```python
from build123d import *

# Parameters (mm, degrees)
BOSS_EXTRUDE2_DEPTH = 5
CUT_EXTRUDE1_DEPTH  = 23.574164436
SKETCH3_W           = 3
SKETCH3_H           = 3.88
BOSS_EXTRUDE3_DEPTH = 12
BOSS_EXTRUDE4_REACH = 35.791
SKETCH4_W           = 3
SKETCH4_H           = 6.078503162
SKETCH6_W           = 3
SKETCH6_H           = 23.7
BOSS_EXTRUDE5_DEPTH = 10.921497
CUT_EXTRUDE2_DEPTH  = 26.634408517
FILLET1_R           = 10
FILLET2_R           = 5


with BuildPart() as part:
    # Sketch1 → Boss-Extrude2 (new body)
    with BuildSketch(Plane(origin=(0, 0, 0), x_dir=(0, 1, 0), z_dir=(0, 0, 1))):
        Polygon((-11.85, 0), (11.85, 0), (11.85, -12.4), (11.85, -15.4), (15.73, -15.4), (15.73, -12.4), (15.73, -0.1), (15.73, 3.9), (-15.73, 3.9), (-15.73, -0.1), (-15.73, -12.4), (-15.73, -15.4), (-11.85, -15.4), (-11.85, -12.4), align=None)
    extrude(amount=BOSS_EXTRUDE2_DEPTH)

    # Sketch2 → Cut-Extrude1 (cut, through all)
    with BuildSketch(Plane.XY.offset(5)):
        with BuildLine():
            Line((4.56, -12.29), (7.06, -12.29))
            ThreePointArc((7.06, -12.29), (8.26, -13.49), (7.06, -14.69))
            Line((7.06, -14.69), (4.56, -14.69))
            ThreePointArc((4.56, -14.69), (3.36, -13.49), (4.56, -12.29))
        make_face()
        with BuildLine():
            Line((4.56, 12.29), (7.06, 12.29))
            ThreePointArc((7.06, 12.29), (8.26, 13.49), (7.06, 14.69))
            Line((7.06, 14.69), (4.56, 14.69))
            ThreePointArc((4.56, 14.69), (3.36, 13.49), (4.56, 12.29))
        make_face()
    extrude(amount=-CUT_EXTRUDE1_DEPTH, mode=Mode.SUBTRACT)

    # Sketch3 → Boss-Extrude3 (add)
    with BuildSketch(Plane(origin=(0, 0, 0), x_dir=(1, 0, 0), z_dir=(0, 0, -1))):
        with Locations((13.9, -13.79)):
            Rectangle(SKETCH3_W, SKETCH3_H)
        with Locations((13.9, 13.79)):
            Rectangle(SKETCH3_W, SKETCH3_H)
    extrude(amount=BOSS_EXTRUDE3_DEPTH)

    # Sketch4 → Boss-Extrude4 (add, up to next)
    with BuildSketch(Plane(origin=(0, -11.85, 0), x_dir=(-1, 0, 0), z_dir=(0, 1, 0)), mode=Mode.PRIVATE) as boss_extrude4_sk1:
        with Locations((-13.9, -8.960748419)):
            Rectangle(SKETCH4_W, SKETCH4_H)
    boss_extrude4_tool1 = extrude(boss_extrude4_sk1.sketch, amount=BOSS_EXTRUDE4_REACH, mode=Mode.PRIVATE) - part.part
    add(boss_extrude4_tool1.solids().sort_by_distance((13.9, -11.85, -8.960748))[0])

    # Sketch6 → Boss-Extrude5 (add)
    with BuildSketch(Plane.XY.offset(-5.921496838)):
        with Locations((13.9, 0)):
            Rectangle(SKETCH6_W, SKETCH6_H)
    extrude(amount=BOSS_EXTRUDE5_DEPTH)

    # Sketch5 → Cut-Extrude2 (cut, through all)
    with BuildSketch(Plane(origin=(12.4, 0, 0), x_dir=(0, -1, 0), z_dir=(-1, 0, 0))):
        with BuildLine():
            Line((0, -6.759630835), (-1.108998315, -7.86862915))
            ThreePointArc((-1.108998315, -7.86862915), (-0.136723769, -10.592070465), (1.355251929, -8.114882764))
            Line((1.355251929, -8.114882764), (0, -6.759630835))
        make_face()
    extrude(amount=-CUT_EXTRUDE2_DEPTH, mode=Mode.SUBTRACT)

    # Fillet1
    fillet1_edges = [part.edges().sort_by_distance(p)[0] for p in [
        (13.9, 15.73, -12),
        (13.9, -15.73, -12),
    ]]
    fillet(fillet1_edges, radius=FILLET1_R)

    # Fillet2
    fillet2_edges = [part.edges().sort_by_distance(p)[0] for p in [
        (-3.9, -15.73, 2.5),
        (-3.9, 15.73, 2.5),
    ]]
    fillet(fillet2_edges, radius=FILLET2_R)


solid = part.part
```
Input: part model. Units: mm. Frame: model coordinates. A direction names the side the tool comes from. Give positions to 0.01 mm unless a question says otherwise; leave off trailing zeros. Order: outer loops, then holes, each group sorted by start corner. A loop starts at its lowest first (then second) coordinate and runs counter-clockwise, first axis right, second up. Notation, with made-up numbers: (82.25, -11.5) - (111.25, -11.5) arc R27 ccw to (111.25, 24.5) - close; hole circle Ø11 at (69.5, -21). An arc over 180 degrees is marked (long way). One line per item, written item: value.
1. Cut plane C-C, the plane x = 0.5. Output: boundary loops of the cut face in (y, z), and give its area (3 significant figures).
Determined:
outline: (-15.69, 0) - (-11.85, 0) - (-11.85, 5) - (-15.69, 5) - close; (11.85, 0) - (15.69, 0) - (15.69, 5) - (11.85, 5) - close
area: 38.4 mm2
2. Reachability of faces 1 (the face through (-2.4, 14.3, 2.5)), 2 (the face through (-3.9, 0, 2)), 3 (the face through (-1, 1, 0)), 4 (the face through (13.88, 0.55, -7.31)), 5 (the face through (6, -11.85, 2)) from +Z, -Z, +X, -X, +Y, -Y: full face, straight path, thin tool, end or side. Return the list, or none.
Determined:
face 1: +Z, -Z, -X, +Y
face 2: +Z, -Z, -X, +Y, -Y
face 3: -Z, -X, +Y, -Y
face 4: +X, -X
face 5: +Z, -Z
3. Draft query along Y for faces 6 (the face through (8, 15.73, 2)), 7 (the face through (14, 0, -12)), 8 (the face through (12.4, 0, -4)). Return one class per face: released by +Y, released by -Y, zero draft, split by the parting line, or undercut.
Determined:
face 6: released by +Y
face 7: zero draft
face 8: undercut
4. Cut plane A-A, the plane z = 1. Output: boundary loops of the cut face in (x, y).
Determined:
outline: (-3.9, -10.73) arc R5 ccw to (1.1, -15.73) - (15.4, -15.73) - (15.4, 15.73) - (1.1, 15.73) arc R5 ccw to (-3.9, 10.73) - close; hole (0, -11.85) - (12.4, -11.85) - (12.4, 11.85) - (0, 11.85) - close; hole (4.56, -14.69) - (7.06, -14.69) arc R1.2 ccw to (7.06, -12.29) - (4.56, -12.29) arc R1.2 ccw to start; hole (4.56, 12.29) - (7.06, 12.29) arc R1.2 ccw to (7.06, 14.69) - (4.56, 14.69) arc R1.2 ccw to start
5. Pin query (flat end, axial travel): pin 1 Ø4 at (y, z) = (3.5, -8.5) entering from -X; pin 2 Ø2 at (x, y) = (4.5, 12.5) entering from -Z; pin 3 Ø8 at (y, z) = (11.5, -2.5) entering from -X; pin 4 Ø2.5 at (y, z) = (-0.02, -9) entering from -X. Return the tip coordinate at first contact, or that it passes through.
Determined:
pin 1: x = 12.4
pin 2: z = 0
pin 3: x = -3.9
pin 4: through
6. Cut plane B-B, the plane y = -2. Output: boundary loops of the cut face in (x, z).
Determined:
outline: (-3.9, 0) - (0, 0) - (0, 5) - (-3.9, 5) - close; (12.4, -12) - (15.4, -12) - (15.4, 5) - (12.4, 5) - close
7. Line query: probe 1 along Y at (x, z) = (6, 4); probe 2 along Y at (x, z) = (9.5, 1.75); probe 3 along X at (y, z) = (3, -2.5). Output: solid intervals per line, ascending.
Determined:
probe 1: -15.73 to -14.69, -12.29 to -11.85, 11.85 to 12.29, 14.69 to 15.73
probe 2: -15.73 to -11.85, 11.85 to 15.73
probe 3: 12.4 to 15.4
8. Cut plane D-D, the plane y = 13.49. Output: boundary loops of the cut face in (x, z), and give its area (3 significant figures).
Determined:
outline: (-3.07, 0) - (3.36, 0) - (3.36, 5) - (-3.07, 5) - close; (8.26, 0) - (12.4, 0) - (12.4, -8.31) - (15.4, -8.31) - (15.4, 5) - (8.26, 5) - close
area: 92.8 mm2
